Print and shaded views of the part. All mm, measured from the part's lowest x, y and z. A direction names the side the tool comes from. Coordinates: 2 decimals unless noted, no trailing zeros. Write each loop counter-clockwise with the first axis right and the second up, starting at its lowest first coordinate (ties: lowest second). Pieces come first, ordered by that corner, then holes. Notation, with made-up numbers: (-29, -4) -> (0, -4) arc R7 ccw to (0, 6) -> close; hole circle Ø6 at (45.25, 54.25). An arc over 180 degrees is marked (long way). Write item = value, one per line.
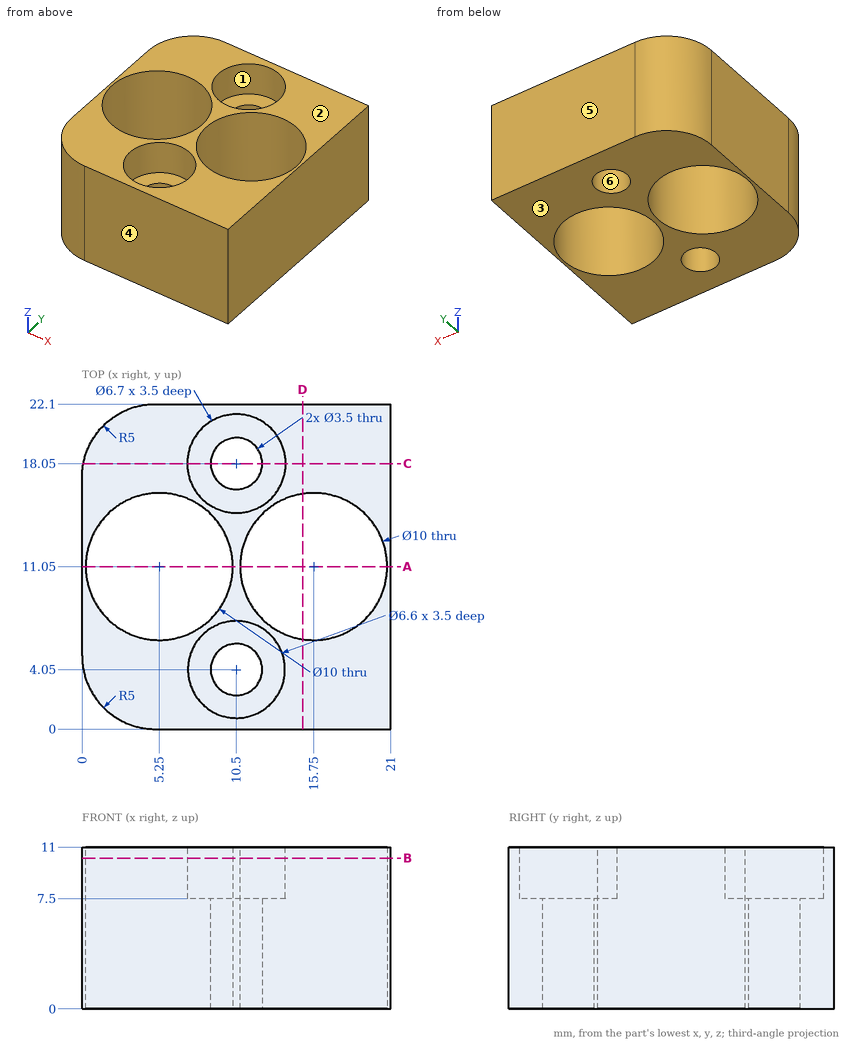
Q1. Pin check, flat tips, straight feed: pin 1 (1.5 mm diameter, centred on x = 17, y = 9, fed in from -Z); pin 2 (3.5 mm diameter, centred on x = 11, y = 3, fed in from +Z). Stop position of each tip, or through.
Model answer:
pin_1 = through
pin_2 = 7.5
Q2. Saw through at C-C on y = 18.05. Give the cut face in (x, z).
Model answer:
outline = (0.09, 0) -> (8.75, 0) -> (8.75, 7.5) -> (7.15, 7.5) -> (7.15, 11) -> (0.09, 11) -> close; (12.25, 0) -> (21, 0) -> (21, 11) -> (13.85, 11) -> (13.85, 7.5) -> (12.25, 7.5) -> close
Q3. Which spindle directions (+Z, -Z, +X, -X, +Y, -Y) get a long thin tool onto all of the face, cutting with end or side? Do the marked faces 1 and 2. Say none if no direction does.
Model answer:
face_1 = +Z
face_2 = +Z, +X, -X, +Y, -Y
Q4. Saw through at B-B on z = 10.25. Give the cut face in (x, y), and give its area (3 significant figures).
Model answer:
outline = (0, 5) arc R5 ccw to (5, 0) -> (21, 0) -> (21, 22.1) -> (5, 22.1) arc R5 ccw to (0, 17.1) -> close; hole circle Ø10 at (5.25, 11.05); hole circle Ø6.7 at (10.5, 18.05); hole circle Ø6.6 at (10.5, 4.05); hole circle Ø10 at (15.75, 11.05)
area = 227 mm²
Q5. Saw through at A-A on y = 11.05. Give the cut face in (x, z).
Model answer:
outline = (0, 0) -> (0.25, 0) -> (0.25, 11) -> (0, 11) -> close; (10.25, 0) -> (10.75, 0) -> (10.75, 11) -> (10.25, 11) -> close; (20.75, 0) -> (21, 0) -> (21, 11) -> (20.75, 11) -> close
Q6. Mould opens along Y. For the marked faces 3, 4, 5 and 6 say: released by +Y, released by -Y, zero draft, split by the parting line, or undercut.
Model answer:
face_3 = zero draft
face_4 = released by -Y
face_5 = released by +Y
face_6 = undercut
Q7. Saw through at D-D on x = 15. Give the cut face in (y, z).
Model answer:
outline = (0, 0) -> (6.11, 0) -> (6.11, 11) -> (0, 11) -> close; (15.99, 0) -> (22.1, 0) -> (22.1, 11) -> (15.99, 11) -> close
Q8. Probe line 1 (Y direction, x = 15.75, z = 2.5); line 2 (X direction, y = 11.5, z = 9.5); line 3 (X direction, y = 8.5, z = 0.75). List the from-to ranges inside material, lowest first. Write a range as from..to.
Model answer:
line_1 = 0..6.05, 16.05..22.1
line_2 = 0..0.27, 10.23..10.77, 20.73..21
line_3 = 0..0.95, 9.55..11.45, 20.05..21
